Work out the finished part from the listing and answer in its coordinate system (mm). Give positions to 0.01 mm unless a question says otherwise; leave off trailing zeros. Loops run counter-clockwise (first coordinate to the right, second up) from the corner with the lowest first, then second, coordinate; pieces in that order, holes last. Notation, with made-up numbers: (43.5, 43.25) - (56.5, 43.25) arc R24 ccw to (56.5, 69.25) - close; hole circle Ø2 at (-35.75, 43). An arc over 180 degrees is marked (long way). One line per question, with ' | ' between items. Start each with the question number.
1. Section B-B (x = 32.5) is taken. Determine the outline of the cut face in (y, z) (3 decimals).
2. Section C-C (y = 1.7) is taken. Determine the outline of the cut face in (x, z).
3. Section A-A (z = 32) is taken. Determine the outline of the cut face in (x, y) (3 decimals), plus the area to 3 significant figures.
4. Find the intervals of material crossed by line 1 (X direction, y = 1.8, z = 54); line 2 (X direction, y = 0.5, z = 2); line 3 (Z direction, x = 67, y = 2.4), in increasing order.
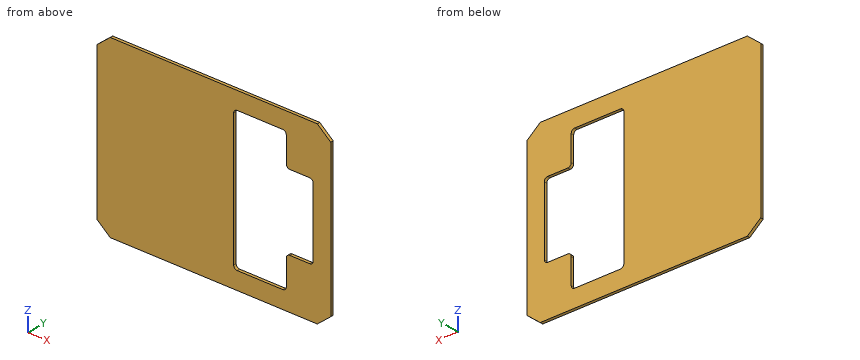
from build123d import *

# Parameters (mm, degrees)
BOSS_EXTRUDE1_DEPTH = 3.175
CUT_EXTRUDE1_DEPTH  = 4.175


with BuildPart() as part:
    # Sketch1 → Boss-Extrude1 (new body)
    with BuildSketch(Plane(origin=(0, 0, 0), x_dir=(1, 0, 0), z_dir=(0, 1, 0))):
        Polygon((127, -83.004896035), (112.406853359, -95.25), (-112.406853359, -95.25), (-127, -83.004896035), (-127, 83.004896035), (-112.406853359, 95.25), (112.406853359, 95.25), (127, 83.004896035), align=None)
    extrude(amount=BOSS_EXTRUDE1_DEPTH)

    # Sketch2 → Cut-Extrude1 (cut, through all)
    with BuildSketch(Plane(origin=(0, 3.175, 0), x_dir=(1, 0, 0), z_dir=(0, 1, 0))):
        with BuildLine():
            Line((82.55, 40.894), (104.14, 40.894))
            ThreePointArc((104.14, 40.894), (106.834076836, 39.778076836), (107.95, 37.084))
            Line((107.95, 37.084), (107.95, -37.084))
            ThreePointArc((107.95, -37.084), (106.834076836, -39.778076836), (104.14, -40.894))
            Line((104.14, -40.894), (82.55, -40.894))
            ThreePointArc((82.55, -40.894), (79.855923164, -42.009923164), (78.74, -44.704))
            Line((78.74, -44.704), (78.74, -72.39))
            ThreePointArc((78.74, -72.39), (77.624076836, -75.084076836), (74.93, -76.2))
            Line((74.93, -76.2), (25.4, -76.2))
            ThreePointArc((25.4, -76.2), (22.705923164, -75.084076836), (21.59, -72.39))
            Line((21.59, -72.39), (21.59, 72.39))
            ThreePointArc((21.59, 72.39), (22.705923164, 75.084076836), (25.4, 76.2))
            Line((25.4, 76.2), (74.93, 76.2))
            ThreePointArc((74.93, 76.2), (77.624076836, 75.084076836), (78.74, 72.39))
            Line((78.74, 72.39), (78.74, 44.704))
            ThreePointArc((78.74, 44.704), (79.855923164, 42.009923164), (82.55, 40.894))
        make_face()
    extrude(amount=-CUT_EXTRUDE1_DEPTH, mode=Mode.SUBTRACT)


solid = part.part
Conclusion:
1) outline: (0, -95.25) - (3.175, -95.25) - (3.175, -76.2) - (0, -76.2) - close; (0, 76.2) - (3.175, 76.2) - (3.175, 95.25) - (0, 95.25) - close
2) outline: (-127, -83) - (-112.41, -95.25) - (112.41, -95.25) - (127, -83) - (127, 83) - (112.41, 95.25) - (-112.41, 95.25) - (-127, 83) - close; hole (21.59, -72.39) arc R3.81 ccw to (25.4, -76.2) - (74.93, -76.2) arc R3.81 ccw to (78.74, -72.39) - (78.74, -44.7) arc R3.81 cw to (82.55, -40.89) - (104.14, -40.89) arc R3.81 ccw to (107.95, -37.08) - (107.95, 37.08) arc R3.81 ccw to (104.14, 40.89) - (82.55, 40.89) arc R3.81 cw to (78.74, 44.7) - (78.74, 72.39) arc R3.81 ccw to (74.93, 76.2) - (25.4, 76.2) arc R3.81 ccw to (21.59, 72.39) - close
3) outline: (-127, 0) - (21.59, 0) - (21.59, 3.175) - (-127, 3.175) - close; (107.95, 0) - (127, 0) - (127, 3.175) - (107.95, 3.175) - close | area: 532 mm²
4) line 1: -127 to 21.59, 78.74 to 127 | line 2: -127 to 21.59, 107.95 to 127 | line 3: -95.25 to -76.2, 76.2 to 95.25
